from build123d import *

# Parameters (mm, degrees)
F1_DEPTH = 914.4
F2_R     = 6.35
F3_DEPTH = 63.501
F4_R     = 19.05
F5_R     = 63.5
F6_DEPTH = 6.35
F7_R     = 6.35
F8_DEPTH = 203.2


with BuildPart() as f1:
    # F0 (on Top) → F1 (new body)
    with BuildSketch(Plane.XY):
        Polygon((50.8, 31.75), (0, 31.75), (0, -31.75), (50.8, -31.75), (50.8, -25.4), (6.35, -25.4), (6.35, 25.4), (50.8, 25.4), align=None)
    extrude(amount=F1_DEPTH)

    # F2 (on face) → F3 (cut, through all)
    with BuildSketch(Plane.XZ.offset(31.75)):
        with Locations((31.75, 901.7)):
            Circle(F2_R)
        with Locations((38.1, 609.6)):
            Circle(F2_R)
    extrude(amount=-F3_DEPTH, mode=Mode.SUBTRACT)

    # F4
    f4_edges = [f1.edges().sort_by_distance(p)[0] for p in [
        (50.8, -28.575, 914.4),
        (50.8, 28.575, 914.4),
    ]]
    fillet(f4_edges, radius=F4_R)

    # F5 (on Top) → F6 (join)
    with BuildSketch(Plane.XY):
        with Locations((25.4, 0)):
            Circle(F5_R)
    extrude(amount=-F6_DEPTH)

    # F7 (on face) → F8 (join)
    with BuildSketch(Plane(origin=(0, 0, -6.35), x_dir=(1, 0, 0), z_dir=(0, 0, -1))):
        with Locations((50.8, 0)):
            Circle(F7_R)
    extrude(amount=F8_DEPTH)


solid = f1.part
Design review of the part built by this model. Coordinates are the model's own, in mm. A direction names the side the tool comes from. Round coordinates to 2 decimals unless told otherwise and drop trailing zeros. Loops run counter-clockwise (first coordinate to the right, second up) from the corner with the lowest first, then second, coordinate; pieces in that order, holes last. Notation, with made-up numbers: (70.5, -8) -> (76.5, -8) arc R22 cw to (76.5, 2) -> close; hole circle Ø7 at (-30.75, -19.5). An arc over 180 degrees is marked (long way). Use one line per item in the form item = value. Start each with the question number.
Q1. Machinability: for faces 1 (the face through (25, -31.75, 451)), 2 (the face through (0, 0, 451)), 3 (the face through (6.35, 0, 451)), 4 (the face through (26, 31.75, 451)), which of the approach directions +Z, -Z, +X, -X, +Y, -Y give a long, thin tool a straight path to every point of the face, cutting with its end or side? Answer none if there is none.
Q2. We need section C-C on y = -43.5. Give the boundary of the cut face in (x, z).
Q3. We need section B-B on x = 71. Give the boundary of the cut face in (y, z), then the cut area to 3 significant figures.
Q4. Draft analysis for pull direction Y (two halves, no side actions). For faces 5 (the face through (28, 25.4, 451)), 6 (the face through (11.63, -61.99, -3.13)), 7 (the face through (25, 1, 0)), 8 (the face through (45.37, 28.62, 908.67)), state which applies: +Y half, -Y half, draft (parallel to the pull), parting line (faces both ways), or undercut.
Q5. For pin 1 Ø22 at (x, z) = (24.5, 258) entering from +Y; pin 2 Ø5 at (x, y) = (48, -11.5) entering from +Z; pin 3 Ø2 at (x, y) = (3.5, 21) entering from -Z, all flat-tipped, find the tip position at first contact; note any pin that passes through.
Q6. Wall thickness on line 1 along Y through (x, z) = (29.5, 461.5); line 2 along X through (y, z) = (28.5, 609.6); line 3 along X through (y, z) = (16.5, 735): over which ranges is each line inside the solid? List them lowest first. Write a range as [from, to].
Q7. We need section D-D on z = -83. Give the boundary of the cut face in (x, y).
Q8. We need section A-A on z = 558. Give the boundary of the cut face in (x, y), then the cut area to 3 significant figures.
Calculated:
q1.face_1 = +Z, +X, -X, -Y
q1.face_2 = +Z, -X, +Y, -Y
q1.face_3 = +Z, +X
q1.face_4 = +Z, +X, -X, +Y
q2.outline = (-20.86, -6.35) -> (71.66, -6.35) -> (71.66, 0) -> (-20.86, 0) -> close
q3.outline = (-44.19, -6.35) -> (44.19, -6.35) -> (44.19, 0) -> (-44.19, 0) -> close
q3.area = 561 mm²
q4.face_5 = undercut
q4.face_6 = parting line
q4.face_7 = undercut
q4.face_8 = draft
q5.pin_1 = 31.75
q5.pin_2 = 0
q5.pin_3 = -6.35
q6.line_1 = [-31.75, -25.4], [25.4, 31.75]
q6.line_2 = [0, 31.75], [44.45, 50.8]
q6.line_3 = [0, 6.35]
q7.outline = circle Ø12.7 at (50.8, 0)
q8.outline = (0, -31.75) -> (50.8, -31.75) -> (50.8, -25.4) -> (6.35, -25.4) -> (6.35, 25.4) -> (50.8, 25.4) -> (50.8, 31.75) -> (0, 31.75) -> close
q8.area = 968 mm²
